```python
from build123d import *

# Parameters (mm, degrees)
F0_W          = 31
F0_H          = 34.5
F1_DEPTH      = 36.5
F3_DEPTH      = 34.5
F5_R          = 6.35
F5_R_2        = 4.6
F6_DEPTH      = 28
F7_W          = 11.7
F7_H          = 13
F7_R          = 1.05
F8_DEPTH      = 3.0000000261
F4_R          = 1.75
F9_DEPTH      = 3.0000000261
F10_DEPTH     = 1.5
F11_DEPTH     = 3.0000000261
F12_R         = 2
F13_T4_DEPTH  = 47.4768176547
F13_T9_DEPTH  = 47.4768176547
F13_T15_DEPTH = 60.4536353093
F13_T21_DEPTH = 47.4768176547
F13_T23_DEPTH = 60.4536353093


# Not quite as in the source:
# - a fillet or chamfer that OpenCascade refuses, or shapes differently, is made with other operations: its cross-section is extruded or revolved along the edge and cut away or added
# - a feature names something its author has since deleted; it is built from what else it names


with BuildPart() as f1:
    # F0 (on Top) → F1 (new body)
    with BuildSketch(Plane.XY):
        Rectangle(F0_W, F0_H)
    extrude(amount=F1_DEPTH)

    # F2 (on face) → F3 (cut, through all)
    with BuildSketch(Plane.XZ.offset(17.25)):
        Polygon((-15.5, 36.5), (-15.5, 3.0000000261), (2.9619937352, 3.0000000261), (12.4999999739, 16.2664996126), (12.4999999739, 36.5), align=None)
        Polygon((15.5, 15.3), (4.5, 0), (15.5, 0), align=None)
    extrude(amount=-F3_DEPTH, mode=Mode.SUBTRACT)

    # F5 (on face) → F6 (join)
    with BuildSketch(Plane.XY.offset(3.0000000261)):
        with Locations((-5.55, 0)):
            Circle(F5_R)
        with Locations((-5.55, 0)):
            Circle(F5_R_2, mode=Mode.SUBTRACT)
    extrude(amount=F6_DEPTH)

    # F7 (on face) → F8 (cut, through all)
    with BuildSketch(Plane.YZ.offset(15.5)):
        with Locations((6.15, 26)):
            Rectangle(F7_W, F7_H)
        with Locations((-6.15, 26)):
            Rectangle(F7_W, F7_H)
        with Locations((-14.3, 26)):
            Circle(F7_R)
        with Locations((14.3, 26)):
            Circle(F7_R)
    extrude(amount=-F8_DEPTH, mode=Mode.SUBTRACT)

    # F4 (on face) → F9 (cut, through all)
    with BuildSketch(Plane.XY.offset(3.0000000261)):
        with Locations((-11.3, -13)):
            Circle(F4_R)
        with Locations((0.2, 13)):
            Circle(F4_R)
    extrude(amount=-F9_DEPTH, mode=Mode.SUBTRACT)

    # F4 (on face) → F10 (cut)
    with BuildSketch(Plane.XY.offset(3.0000000261)):
        Polygon((-14.3, -11.2679491924), (-14.3, -14.7320508076), (-11.3, -16.4641016151), (-8.3, -14.7320508076), (-8.3, -11.2679491924), (-11.3, -9.5358983849), align=None)
        with Locations((-11.3, -13)):
            Circle(F4_R, mode=Mode.SUBTRACT)
        Polygon((0.2, 16.4641016151), (-2.8, 14.7320508076), (-2.8, 11.2679491924), (0.2, 9.5358983849), (2.9619937352, 11.1305362114), (2.9619937352, 14.8694637886), align=None)
        with Locations((0.2, 13)):
            Circle(F4_R, mode=Mode.SUBTRACT)
    extrude(amount=-F10_DEPTH, mode=Mode.SUBTRACT)

    # F5 (on face) → F11 (cut, through all)
    with BuildSketch(Plane.XY.offset(3.0000000261)):
        with Locations((-5.55, 0)):
            Circle(F5_R_2)
    extrude(amount=-F11_DEPTH, mode=Mode.SUBTRACT)

    # F12
    f12_edges = [f1.edges().sort_by_distance(p)[0] for p in [
        (14, -17.25, 36.5),
        (14, 17.25, 36.5),
    ]]
    fillet(f12_edges, radius=F12_R)

    # F13: chamfer of 5 on 2 edges, made by hand


with BuildPart() as f13_tool2:
    # F13_s3 → F13_t4 (new body)
    with BuildSketch(Plane.XZ.offset(17.25)):
        Polygon((12.4999999739, 21.2664996126), (9.5812730216, 12.2068157607), (12.4999999739, 16.2664996126), align=None)
    extrude(amount=-F13_T4_DEPTH)

    split(bisect_by=Plane.XZ.offset(12), keep=Keep.TOP)


with BuildPart() as f1_1:
    add(f1.part)

    # F13_t1: union F13_tool2
    add(f13_tool2.part)


with BuildPart() as f13_tool7:
    # F13_s8 → F13_t9 (new body)
    with BuildSketch(Plane.XZ.offset(30.2268176547)):
        Polygon((12.4999999739, 21.2664996126), (9.5812730216, 12.2068157607), (12.4999999739, 16.2664996126), align=None)
    extrude(amount=-F13_T9_DEPTH)

    split(bisect_by=Plane.XY.offset(19.5), keep=Keep.BOTTOM)

    split(bisect_by=Plane.XZ.offset(12), keep=Keep.BOTTOM)


with BuildPart() as f1_2:
    add(f1_1.part)

    # F13_t6: union F13_tool7
    add(f13_tool7.part)


with BuildPart() as f13_tool13:
    # F13_s14 → F13_t15 (new body)
    with BuildSketch(Plane.XZ.offset(30.2268176547)):
        Polygon((12.4999999739, 21.2664996126), (9.5812730216, 12.2068157607), (12.4999999739, 16.2664996126), align=None)
    extrude(amount=-F13_T15_DEPTH)

    split(bisect_by=Plane.XZ.offset(-0.3), keep=Keep.TOP)

    split(bisect_by=Plane.XZ.offset(0.3), keep=Keep.BOTTOM)


with BuildPart() as f1_3:
    add(f1_2.part)

    # F13_t12: union F13_tool13
    add(f13_tool13.part)


with BuildPart() as f13_tool19:
    # F13_s20 → F13_t21 (new body)
    with BuildSketch(Plane.XZ.offset(30.2268176547)):
        Polygon((12.4999999739, 21.2664996126), (9.5812730216, 12.2068157607), (12.4999999739, 16.2664996126), align=None)
    extrude(amount=-F13_T21_DEPTH)

    split(bisect_by=Plane.XZ.offset(-12), keep=Keep.BOTTOM)


with BuildPart() as f1_4:
    add(f1_3.part)

    # F13_t18: union F13_tool19
    add(f13_tool19.part)

    # F13_s24 → F13_t23 (cut)
    with BuildSketch(Plane.XZ.offset(-30.2268176547)):
        Polygon((15.5, 20.3), (12.5812730476, 11.2403161481), (15.5, 15.3), align=None)
    extrude(amount=F13_T23_DEPTH, mode=Mode.SUBTRACT)


solid = f1_4.part
```
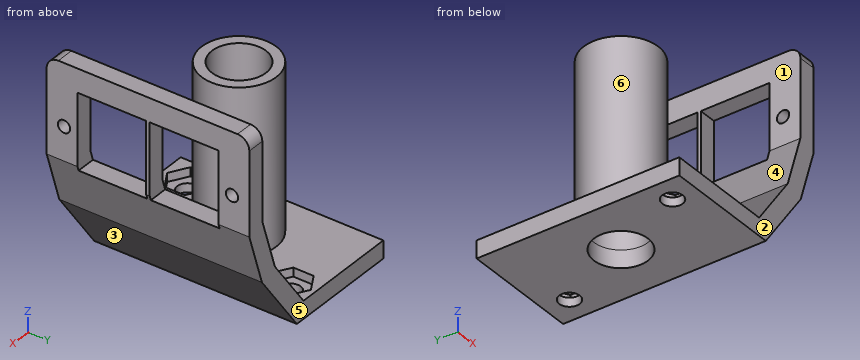
Verification items for the finished model (mm, model axes). Face numbers are marked on the shaded views. A direction names the side the tool comes from. Round coordinates to 2 decimals unless told otherwise and drop trailing zeros. Write each loop counter-clockwise with the first axis right and the second up, starting at its lowest first coordinate (ties: lowest second). Pieces come first, ordered by that corner, then holes. Notation, with made-up numbers: (59, 31) - (89, 31) arc R19 ccw to (89, 52) - close; hole circle Ø3 at (8, -9). An arc over 180 degrees is marked (long way). Answer as a JSON object with one key per item and string values. Group by question number.
Q1. Section check C-C, the plane x = -5.55. Enter the section's corners in (y, z), plus the area to 3 significant figures.
Q2. Go/stop test with flat-tipped pins: pin 1 Ø1.6 at (y, z) = (-12.5, 2.5) entering from +X; pin 2 Ø4 at (x, z) = (8.5, 20.5) entering from -Y; pin 3 Ø12 at (y, z) = (-4.5, 31) entering from -X; pin 4 Ø10 at (x, y) = (-5.5, -9) entering from +Z. Record where each tip stops, or that it passes through.
Q3. Section check A-A, the plane z = 23. Enter the section's corners in (x, y).
Q4. Tool access check on the marked faces 1 and 2. Record the directions out of +Z, -Z, +X, -X, +Y, -Y that give a thin tool (end or side, any length) a straight path to the whole face; none if there is none.
Q5. Thickness scan on line 1 (X direction, y = 4, z = 17); line 2 (Y direction, x = -11.3, z = 0.5); line 3 (X direction, y = 2, z = 13.5). Record the ranges inside material, lowest first.
Q6. Mould release check, pull along X, two halves, no side actions. Record for the marked faces 3, 4, 5 and 6: released by +X, released by -X, zero draft, split by the parting line, or undercut.
Q7. Section check B-B, the plane y = 8.5. Enter the section's corners in (x, z).
Q8. Section check D-D, the plane z = 19. Enter the section's corners in (x, y).
Found:
{
 "1": {"outline": "(-17.25, 0) - (-4.6, 0) - (-4.6, 31) - (-6.35, 31) - (-6.35, 3) - (-17.25, 3) - close; (4.6, 0) - (17.25, 0) - (17.25, 3) - (6.35, 3) - (6.35, 31) - (4.6, 31) - close", "area": "174 mm^2"},
 "2": {"pin 1": "stops at x = 6.87", "pin 2": "passes through", "pin 3": "stops at x = -11.9", "pin 4": "stops at z = 31"},
 "3": {"outline": "circle Ø12.7 at (-5.55, 0); (12.5, -17.25) - (15.5, -17.25) - (15.5, -12) - (12.5, -12) - close; (12.5, -0.3) - (15.5, -0.3) - (15.5, 0.3) - (12.5, 0.3) - close; (12.5, 12) - (15.5, 12) - (15.5, 17.25) - (12.5, 17.25) - close; hole circle Ø9.2 at (-5.55, 0)"},
 "4": {"face 1": "+Z, +Y, -Y", "face 2": "+Z, -Z, +X, -X, -Y"},
 "5": {"line 1": "x = -10.48 to -7.82, -3.28 to -0.62, 11.13 to 14.44", "line 2": "y = -17.25 to -14.75, -11.25 to 17.25", "line 3": "x = -11.58 to -9.69, -1.41 to 0.48, 10 to 13.31"},
 "6": {"face 3": "released by +X", "face 4": "undercut", "face 5": "zero draft", "face 6": "undercut"},
 "7": {"outline": "(-15.5, 0) - (4.5, 0) - (12.58, 11.24) - (15.24, 19.5) - (11.93, 19.5) - (9.58, 12.21) - (2.96, 3) - (-15.5, 3) - close; (12.5, 32.5) - (15.5, 32.5) - (15.5, 36.5) - (12.5, 36.5) - close"},
 "8": {"outline": "circle Ø12.7 at (-5.55, 0); (11.77, -17.25) - (15.08, -17.25) - (15.08, 17.25) - (11.77, 17.25) - close; hole circle Ø9.2 at (-5.55, 0)"}
}
